Answer from the drawing. Dimensions are ordinates in mm from the lowest x, y and z of the part. Coordinates: 2 decimals unless noted, no trailing zeros. Write each loop counter-clockwise with the first axis right and the second up, starting at its lowest first coordinate (ties: lowest second). Pieces come first, ordered by that corner, then holes. Notation, with made-up numbers: (74, 55.25) -> (124, 55.25) arc R16 cw to (124, 68.25) -> close; hole circle Ø5 at (-12.5, 5). An arc over 180 degrees is marked (long way). One line per item, written item: value. Start each with the question number.
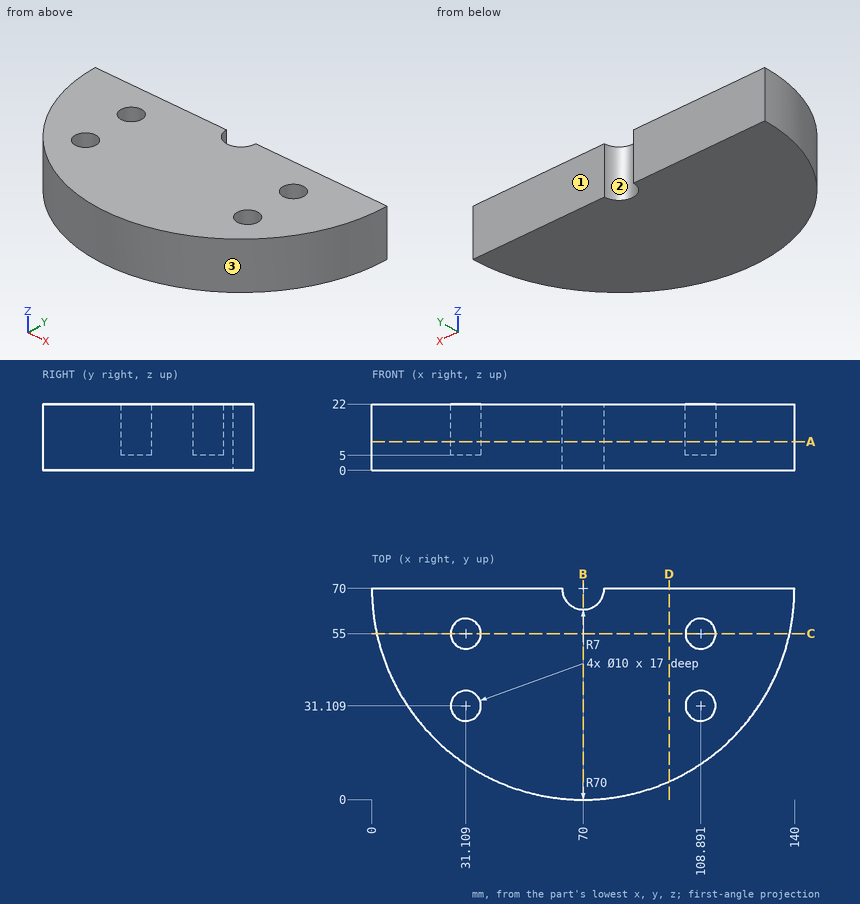
1. A cutting plane is placed at B-B on x = 70. Give the vertices of the cut face in (y, z), then the cut area to 3 significant figures.
2. A cutting plane is placed at D-D on x = 98.5. Give the vertices of the cut face in (y, z).
3. Given pin 1 (3 mm diameter, centred on x = 123.5, z = 13, fed in from -Y); pin 2 (3 mm diameter, centred on x = 32.5, y = 33.5, fed in from +Z); pin 3 (5 mm diameter, centred on y = 29, z = 17.5, fed in from +X), each flat-ended and moving along its own axis, determine where each tip first touches the part or whether it passes through.
4. Find the intervals of material crossed by probe 1 along Y at (x, z) = (29, 14.5); probe 2 along X at (y, z) = (29, 20.5); probe 3 along X at (y, z) = (33.5, 8.5), in increasing order. Write a range as from..to.
5. A cutting plane is placed at C-C on y = 55. Give the vertices of the cut face in (x, z).
6. A cutting plane is placed at A-A on z = 9.5. Give the vertices of the cut face in (x, y), then the cut area to 3 significant figures.
7. For a pull along X with two mould halves and no side action, classify the marked faces 1, 2 and 3 as +X half, -X half, draft (parallel to the pull), parting line (faces both ways), or undercut.
Derived:
1. outline: (0, 0) -> (63, 0) -> (63, 22) -> (0, 22) -> close
1. area: 1,390 mm2
2. outline: (6.06, 0) -> (70, 0) -> (70, 22) -> (6.06, 22) -> close
3. pin 1: stops at y = 23.14
3. pin 2: stops at z = 5
3. pin 3: stops at x = 128.46
4. probe 1: y = 13.26..26.58, 35.64..50.47, 59.53..70
4. probe 2: x = 13.26..26.58, 35.64..104.36, 113.42..126.74
4. probe 3: x = 10.27..26.72, 35.5..104.5, 113.28..129.73
5. outline: (1.63, 0) -> (138.37, 0) -> (138.37, 22) -> (113.89, 22) -> (113.89, 5) -> (103.89, 5) -> (103.89, 22) -> (36.11, 22) -> (36.11, 5) -> (26.11, 5) -> (26.11, 22) -> (1.63, 22) -> close
6. outline: (0, 70) arc R70 ccw to (140, 70) -> (77, 70) arc R7 cw to (63, 70) -> close; hole circle Ø10 at (31.11, 31.11); hole circle Ø10 at (31.11, 55); hole circle Ø10 at (108.89, 31.11); hole circle Ø10 at (108.89, 55)
6. area: 7,310 mm2
7. face 1: draft
7. face 2: undercut
7. face 3: parting line
